from build123d import *

# Parameters (mm, degrees)
SKETCH1_R      = 1.3
EXTRUDE1_DEPTH = 3


with BuildPart() as part:
    # Sketch1 → Extrude1 (new body)
    with BuildSketch(Plane.XY):
        Polygon((70, -179.753959847), (-15, -179.753959847), (-25, -169.753959847), (-25, -79.753959847), (-10, -64.753959847), (-10, 24.003545781), (0, 34.003545781), (54.5, 34.003545781), (42.5, 22.003545781), (4.970562749, 22.003545781), (2, 19.032983033), (2, -69.724522596), (-13, -84.724522596), (-13, -164.783397099), (-10.029437251, -167.753959847), (58, -167.753959847), align=None)
        with Locations((-4, 14.243545781)):
            Circle(SKETCH1_R, mode=Mode.SUBTRACT)
    extrude(amount=EXTRUDE1_DEPTH)


solid = part.part
For this review, take the finished solid that the model builds, in its own axes (mm). A direction names the side the tool comes from. Coordinates: 2 decimals unless noted, no trailing zeros. Loops run counter-clockwise (first coordinate to the right, second up) from the corner with the lowest first, then second, coordinate; pieces in that order, holes last. Notation, with made-up numbers: (10, -37.5) - (59, -37.5) arc R24 cw to (59, -1.5) - close; hole circle Ø10 at (9, -7). An arc over 180 degrees is marked (long way). Use a Markdown table: item, result. Add a question column.
Item 1: We need section D-D (y = -22.5). Give the boundary of the cut face in (x, z), and give its area (3 significant figures).
Item 2: We need section C-C (z = 2.3). Give the boundary of the cut face in (x, y).
Item 3: We need section A-A (x = 44.5). Give the boundary of the cut face in (y, z), and give its area (3 significant figures).
Item 4: We need section B-B (x = 22). Give the boundary of the cut face in (y, z).
Item 5: Insertion check: pin 1 Ø1 at (y, z) = (-61, 0.5) entering from -X; pin 2 Ø2 at (x, y) = (-4, 14.24) entering from -Z; pin 3 Ø0.9 at (y, z) = (-130.5, 2) entering from +X. Each pin has a flat end and moves straight along its axis. Give the tip position at first contact, or say it passes through.
Item 6: Tool access review of faces 1 (the face through (-5.395, -77.12, 1.479)), 2 (the face through (63.916, -173.67, 1.479)): name each direction out of +Z, -Z, +X, -X, +Y, -Y from which nothing blocks a thin tool from reaching the whole face with its end or side.
Item 7: Mouldability with a two-part tool opening along Y and no side actions: class faces 3 (the face through (48.584, 28.088, 1.479)), 4 (the face through (-5.07, 28.934, 1.479)), 5 (the face through (1.6, -64.5, 3)) as pulls with the +Y half, pulls with the -Y half, needs draft (parallel to the pull), parting line crosses it, or undercut.
Item 8: For line 1 (Y direction, x = 24, z = 1.1); line 2 (Y direction, x = -4, z = 0.95); line 3 (X direction, y = 15, z = 0.9), list the stretches that pass through material, from the lowest coordinate up.
Results list:
| question | item | result |
|---|---|---|
| 1 | outline | (-10, 0) - (2, 0) - (2, 3) - (-10, 3) - close |
| 1 | area | 36.0 mm^2 |
| 2 | outline | (-25, -169.75) - (-15, -179.75) - (70, -179.75) - (58, -167.75) - (-10.03, -167.75) - (-13, -164.78) - (-13, -84.72) - (2, -69.72) - (2, 19.03) - (4.97, 22) - (42.5, 22) - (54.5, 34) - (0, 34) - (-10, 24) - (-10, -64.75) - (-25, -79.75) - close; hole circle Ø2.6 at (-4, 14.24) |
| 3 | outline | (-179.75, 0) - (-167.75, 0) - (-167.75, 3) - (-179.75, 3) - close; (24, 0) - (34, 0) - (34, 3) - (24, 3) - close |
| 3 | area | 66.0 mm^2 |
| 4 | outline | (-179.75, 0) - (-167.75, 0) - (-167.75, 3) - (-179.75, 3) - close; (22, 0) - (34, 0) - (34, 3) - (22, 3) - close |
| 5 | pin 1 | stops at x = -10 |
| 5 | pin 2 | passes through |
| 5 | pin 3 | stops at x = -13 |
| 6 | face 1 | +Z, -Z, +X |
| 6 | face 2 | +Z, -Z, +X, +Y |
| 7 | face 3 | undercut |
| 7 | face 4 | pulls with the +Y half |
| 7 | face 5 | needs draft |
| 8 | line 1 | y = -179.75 to -167.75, 22 to 34 |
| 8 | line 2 | y = -179.75 to -167.75, -75.72 to 12.94, 15.54 to 30 |
| 8 | line 3 | x = -10 to -5.06, -2.94 to 2 |
